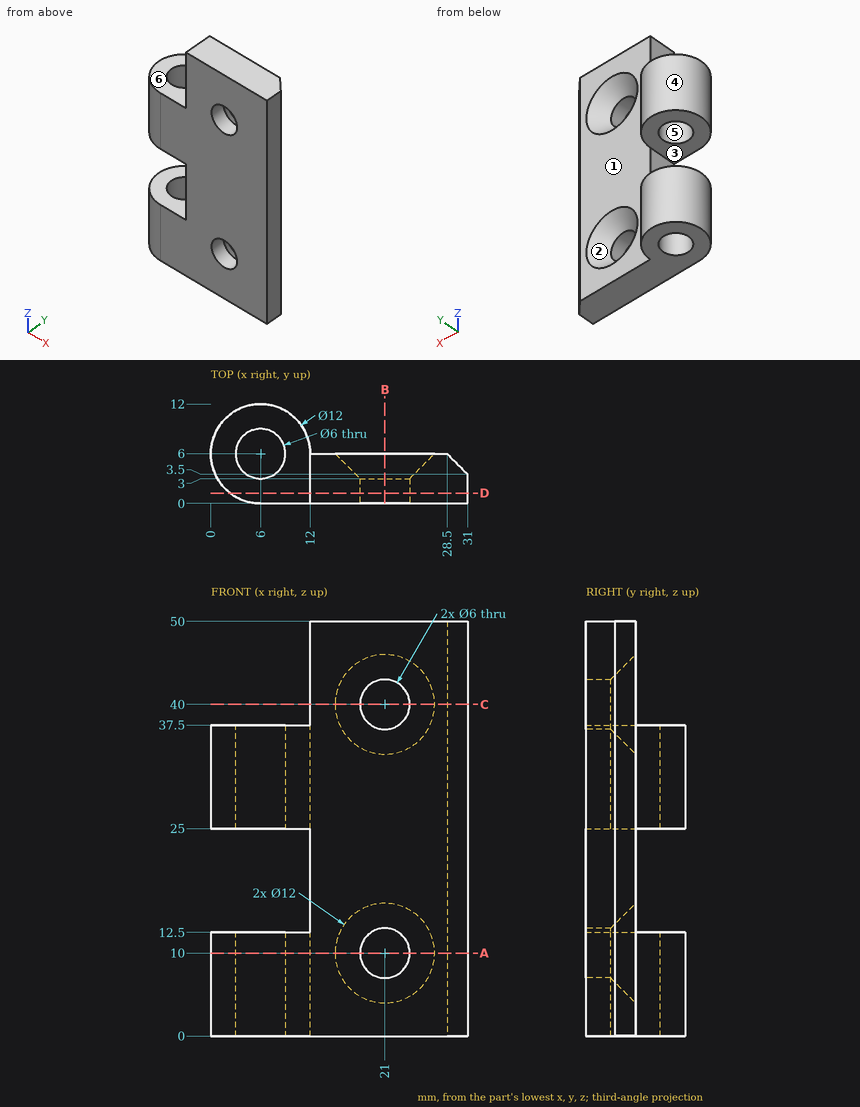
For this review, use the dimensioned drawing (mm, ordinates from the lowest corner) and the shaded views. A direction names the side the tool comes from. Round coordinates to 2 decimals unless told otherwise and drop trailing zeros. Write each loop counter-clockwise with the first axis right and the second up, starting at its lowest first coordinate (ties: lowest second). Pieces come first, ordered by that corner, then holes. Notation, with made-up numbers: (-10, 22) -> (5, 22) arc R31 cw to (5, 48) -> close; hole circle Ø8 at (47, 38). An arc over 180 degrees is marked (long way). One line per item, written item: value. Start each with the question number.
Q1. The part is to be moulded in two halves that separate along Y. For the marked faces 4, 5 and 6, say which applies: pulls with the +Y half, pulls with the -Y half, needs draft (parallel to the pull), parting line crosses it, or undercut.
Q2. Add section B-B (x = 21). Give the boundary of the cut face in (y, z), then the cut area to 3 significant figures.
Q3. Insertion check: P1, Ø8, axis at x = 20, z = 22, coming from the +Y side; P2, Ø7, axis at x = 21, z = 40, coming from the +Y side; P3, Ø5, axis at y = 2, z = 20, coming from the -X side; P4, Ø5, axis at x = 6, y = 6, coming from the +Z side. Each pin has a flat end and moves straight along its axis. Give the tip position at first contact, or say it passes through.
Q4. Add section A-A (z = 10). Give the boundary of the cut face in (x, y).
Q5. Add section C-C (z = 40). Give the boundary of the cut face in (x, y).
Q6. To check wall thickness, follow probe 1 along Z at (x, y) = (21, 1.4); probe 2 along Z at (x, y) = (2.5, 8.25); probe 3 along X at (y, z) = (1.3, 40). State the ranges of each line that lie inside material, in increasing order.
Q7. Tool access review of the marked faces 1, 2 and 3: name each direction out of +Z, -Z, +X, -X, +Y, -Y from which nothing blocks a thin tool from reaching the whole face with its end or side.
Q8. Add section D-D (y = 1.25). Give the boundary of the cut face in (x, z), then the cut area to 3 significant figures.
Response:
1. face 4: parting line crosses it
1. face 5: undercut
1. face 6: needs draft
2. outline: (0, 0) -> (6, 0) -> (6, 4) -> (3, 7) -> (0, 7) -> close; (0, 13) -> (3, 13) -> (6, 16) -> (6, 34) -> (3, 37) -> (0, 37) -> close; (0, 43) -> (3, 43) -> (6, 46) -> (6, 50) -> (0, 50) -> close
2. area: 210 mm^2
3. P1: stops at y = 6
3. P2: stops at y = 3.5
3. P3: stops at x = 12
3. P4: passes through
4. outline: (6, 0) -> (18, 0) -> (18, 3) -> (15, 6) -> (12, 6) arc R6 ccw (long way) to start; (24, 0) -> (31, 0) -> (31, 3.5) -> (28.5, 6) -> (27, 6) -> (24, 3) -> close; hole circle Ø6 at (6, 6)
5. outline: (12, 0) -> (18, 0) -> (18, 3) -> (15, 6) -> (12, 6) -> close; (24, 0) -> (31, 0) -> (31, 3.5) -> (28.5, 6) -> (27, 6) -> (24, 3) -> close
6. probe 1: z = 0 to 7, 13 to 37, 43 to 50
6. probe 2: z = 0 to 12.5, 25 to 37.5
6. probe 3: x = 12 to 18, 24 to 31
7. face 1: +Z, -Z, +X, +Y
7. face 2: +Y
7. face 3: -X, +Y, -Y
8. outline: (2.33, 0) -> (31, 0) -> (31, 50) -> (12, 50) -> (12, 37.5) -> (2.33, 37.5) -> (2.33, 25) -> (12, 25) -> (12, 12.5) -> (2.33, 12.5) -> close; hole circle Ø6 at (21, 10); hole circle Ø6 at (21, 40)
8. area: 1,140 mm^2
